Read the model definition and answer for the solid it produces. Units are mm, in the model's axes. A direction names the side the tool comes from. Round coordinates to 2 decimals unless told otherwise and drop trailing zeros. Answer as a JSON object with one key per item and string values. Group by question number.
Item 1: Consider probe 1 along Z at (x, y) = (54.5, 65); probe 2 along Z at (x, y) = (30, 11); probe 3 along X at (y, z) = (38.5, -40). Determine where each line is inside the solid, lowest interval first. Write a range as from..to.
Item 2: For faces 1 (the flat face through (2, 86, -43)), 2 (the flat face through (3, 46, -43)), determine the directions among +Z, -Z, +X, -X, +Y, -Y from which every point of the face is accessible in a straight line to the end or side of a thin tool.
Item 3: The mould has two halves that part along Z. Classify faces 3 (the cylindrical face through (7.811, 44.933, -7.563)), 4 (the flat face through (44, 0, -43)): pulls with the +Z half, pulls with the -Z half, needs draft (parallel to the pull), parting line crosses it, or undercut.
Item 4: Given P1, Ø14.5, axis at x = 41.5, y = 63, coming from the +Z side; P2, Ø5, axis at y = 47, z = -63, coming from the -X side; P3, Ø1.5, axis at x = 14.5, z = -25.5, coming from the +Y side, each flat-ended and moving along its own axis, determine where each tip first touches the part or whether it passes through.
from build123d import *

# Parameters (mm, degrees)
SKETCH5_W          = 80
SKETCH5_H          = 80
CUT_EXTRUDE1_DEPTH = 81
FILLET1_R          = 16


with BuildPart() as part:
    # Sketch4 → Loft1 section 0
    with BuildSketch(Plane(origin=(0, 86, -86), x_dir=(1, 0, 0), z_dir=(0, 1, 0))):
        with BuildLine():
            Line((88, 2), (88, -88))
            Line((88, -88), (-2, -88))
            Line((-2, -88), (-2, 2))
            Line((-2, 2), (88, 2))
        make_face()
    # Sketch2 → Loft1 section 1
    with BuildSketch(Plane(origin=(0, 0, 0), x_dir=(1, 0, 0), z_dir=(0, 1, 0))):
        with BuildLine():
            Line((0, 0), (86, 0))
            Line((86, 0), (86, 86))
            Line((86, 86), (0, 86))
            Line((0, 86), (0, 0))
        make_face()
    loft()

    # Sketch5 → Cut-Extrude1 (cut)
    with BuildSketch(Plane(origin=(0, 86, 0), x_dir=(1, 0, 0), z_dir=(0, 1, 0))):
        with Locations((43, 43)):
            Rectangle(SKETCH5_W, SKETCH5_H)
    extrude(amount=-CUT_EXTRUDE1_DEPTH, mode=Mode.SUBTRACT)

    # Fillet1
    fillet1_edges = [part.edges().sort_by_distance(p)[0] for p in [
        (87, 43, -87),
        (83, 45.5, -83),
        (87, 43, 1),
        (83, 45.5, -3),
        (-1, 43, 1),
        (3, 45.5, -3),
        (-1, 43, -87),
        (3, 45.5, -83),
    ]]
    fillet(fillet1_edges, radius=FILLET1_R)


solid = part.part
Values found:
{
 "1": {"probe 1": "-87.51..-83, -3..1.51", "probe 2": "-86.26..-83, -3..0.26", "probe 3": "-0.9..3, 83..86.9"},
 "2": {"face 1": "+Z, -Z, +X, -X, +Y", "face 2": "+Y"},
 "3": {"face 3": "undercut", "face 4": "needs draft"},
 "4": {"P1": "z = 1.63", "P2": "x = -1.15", "P3": "y = 5"}
}
